from build123d import *

# Parameters (mm, degrees)
SKETCH_1_W          = 44
SKETCH_1_H          = 81
EXTRUDE_1_DEPTH     = 2
SKETCH_12_W         = 12.5
SKETCH_12_H         = 18.4
CUT_EXTRUDE_3_DEPTH = 7.5
SKETCH_15_W         = 1.5
SKETCH_15_H         = 12
EXTRUDE_10_DEPTH    = 8.8
EXTRUDE_11_DEPTH    = 12
EXTRUDE_12_DEPTH    = 12
FILLET_2_R          = 2
FILLET_3_R          = 2
SKETCH_19_R         = 0.85
CUT_EXTRUDE_4_DEPTH = 12
SKETCH_20_R         = 2
CUT_EXTRUDE_5_DEPTH = 1


with BuildPart() as part:
    # 草图1 → 凸台-拉伸1 (new body)
    with BuildSketch(Plane(origin=(0, 0, 0), x_dir=(1, 0, 0), z_dir=(0, 1, 0))):
        with Locations((0, 2.5)):
            Rectangle(SKETCH_1_W, SKETCH_1_H)
    extrude(amount=EXTRUDE_1_DEPTH)

    # 草图12 → 切除-拉伸3 (cut)
    with BuildSketch(Plane.XZ):
        with Locations((9.849848709, 0)):
            Rectangle(SKETCH_12_W, SKETCH_12_H)
    extrude(amount=-CUT_EXTRUDE_3_DEPTH, mode=Mode.SUBTRACT)

    # 草图15 → 凸台-拉伸10 (add)
    with BuildSketch(Plane(origin=(0, 2, 0), x_dir=(1, 0, 0), z_dir=(0, 1, 0))):
        with Locations((2.849848709, 0)):
            Rectangle(SKETCH_15_W, SKETCH_15_H)
        with Locations((16.849848709, 0)):
            Rectangle(SKETCH_15_W, SKETCH_15_H)
    extrude(amount=EXTRUDE_10_DEPTH)

    # 草图16 → 凸台-拉伸11 (add)
    with BuildSketch(Plane.XY.offset(6)):
        Polygon((3.599848709, 10.8), (5.099848709, 8.3), (3.599848709, 8.3), align=None)
    extrude(amount=-EXTRUDE_11_DEPTH)

    # 草图18 → 凸台-拉伸12 (add)
    with BuildSketch(Plane.XY.offset(6)):
        Polygon((16.099848709, 10.8), (14.599848709, 8.3), (16.099848709, 8.3), align=None)
    extrude(amount=-EXTRUDE_12_DEPTH)

    # 圆角2
    fillet_2_edges = [part.edges().sort_by_distance(p)[0] for p in [
        (2.849848709, 2, -6),
        (2.099848709, 2, 0),
        (2.849848709, 2, 6),
        (16.849848709, 2, -6),
        (16.849848709, 2, 6),
        (17.599848709, 2, 0),
    ]]
    fillet(fillet_2_edges, radius=FILLET_2_R)

    # 圆角3
    fillet_3_edges = [part.edges().sort_by_distance(p)[0] for p in [
        (-22, 1, -43),
        (22, 1, -43),
        (22, 1, 38),
        (-22, 1, 38),
    ]]
    fillet(fillet_3_edges, radius=FILLET_3_R)

    # 草图19 → 切除-拉伸4 (cut)
    with BuildSketch(Plane(origin=(0, 2, 0), x_dir=(1, 0, 0), z_dir=(0, 1, 0))):
        with Locations(Location((-19, 40, 0), (0, 0, 270))):
            Circle(SKETCH_19_R)
        with Locations(Location((19, 40, 0), (0, 0, 270))):
            Circle(SKETCH_19_R)
        with Locations(Location((19, -35, 0), (0, 0, 270))):
            Circle(SKETCH_19_R)
        with Locations(Location((-19, -35, 0), (0, 0, 270))):
            Circle(SKETCH_19_R)
    extrude(amount=-CUT_EXTRUDE_4_DEPTH, mode=Mode.SUBTRACT)

    # 草图20 → 切除-拉伸5 (cut)
    with BuildSketch(Plane.XZ):
        with Locations(Location((-19, 35, 0), (0, 0, 270))):
            Circle(SKETCH_20_R)
        with Locations(Location((19, 35, 0), (0, 0, 270))):
            Circle(SKETCH_20_R)
        with Locations(Location((-19, -40, 0), (0, 0, 270))):
            Circle(SKETCH_20_R)
        with Locations(Location((19, -40, 0), (0, 0, 270))):
            Circle(SKETCH_20_R)
    extrude(amount=-CUT_EXTRUDE_5_DEPTH, mode=Mode.SUBTRACT)


solid = part.part
Verification items for the finished model (mm, model axes). A direction names the side the tool comes from. Round coordinates to 2 decimals unless told otherwise and drop trailing zeros. Loops run counter-clockwise (first coordinate to the right, second up) from the corner with the lowest first, then second, coordinate; pieces in that order, holes last. Notation, with made-up numbers: (27.5, 40.25) - (86.5, 40.25) arc R30 ccw to (86.5, 74.25) - close; hole circle Ø3 at (77, 9.25). An arc over 180 degrees is marked (long way). Write item = value, one per line.
Q1. Depth check by flat-ended pin: pin 1 (0.9 mm diameter, centred on x = 16.5, y = 8.5, fed in from +Z); pin 2 (2.5 mm diameter, centred on x = 4, y = 6, fed in from -Z); pin 3 (2.5 mm diameter, centred on x = -19, z = 35, fed in from -Y). Enter the tip coordinate at first touch or a pass-through.
Here are the results:
pin_1 = 6
pin_2 = -6
pin_3 = 1
Q2. Sectioned sample at D-D on y = 3. Record the boundary of the cut face in (x, z), plus the area to 3 significant figures.
Here are the results:
outline = (1.83, -6.27) - (3.6, -6.27) - (3.6, 6.27) - (1.83, 6.27) - close; (16.1, -6.27) - (17.87, -6.27) - (17.87, 6.27) - (16.1, 6.27) - close
area = 44.3 mm^2
Q3. Tool access check on faces 1 (the flat face through (4, 8.3, 0)), 2 (the flat face through (4.34, 9.57, 0.08)), 3 (the flat face through (10, 1, -9.2)). Record the directions out of +Z, -Z, +X, -X, +Y, -Y that give a thin tool (end or side, any length) a straight path to the whole face; none if there is none.
Here are the results:
face_1 = +Z, -Z, -Y
face_2 = +Z, -Z, +Y
face_3 = +Y, -Y
Q4. Material ranges on L1, parallel to X at y = 0.5, z = -40; L2, parallel to X at y = 1.45, z = -40; L3, parallel to X at y = 1.25, z = 5, recorded low to high.
Here are the results:
L1 = -22 to -21, -17 to 17, 21 to 22
L2 = -22 to -19.85, -18.15 to 18.15, 19.85 to 22
L3 = -22 to 3.6, 16.1 to 22
Q5. Sectioned sample at A-A on x = 7. Record the boundary of the cut face in (y, z), plus the area to 3 significant figures.
Here are the results:
outline = (0, -43) - (2, -43) - (2, -9.2) - (0, -9.2) - close; (0, 9.2) - (2, 9.2) - (2, 38) - (0, 38) - close
area = 125 mm^2
Q6. Sectioned sample at B-B on z = -40. Record the boundary of the cut face in (x, y), plus the area to 3 significant figures.
Here are the results:
outline = (-22, 0) - (-21, 0) - (-21, 1) - (-19.85, 1) - (-19.85, 2) - (-22, 2) - close; (-18.15, 1) - (-17, 1) - (-17, 0) - (17, 0) - (17, 1) - (18.15, 1) - (18.15, 2) - (-18.15, 2) - close; (19.85, 1) - (21, 1) - (21, 0) - (22, 0) - (22, 2) - (19.85, 2) - close
area = 76.6 mm^2
Q7. Mould release check, pull along Z, two halves, no side actions. Record for faces 4 (the cylindrical face through (-17.017, 0.493, -39.74)), 5 (the flat face through (0, 0, -3)), 6 (the flat face through (3, 7, 6)): +Z half, -Z half, draft (parallel to the pull), parting line (faces both ways), or undercut.
Here are the results:
face_4 = undercut
face_5 = draft
face_6 = +Z half
Q8. Sectioned sample at C-C on x = -19. Record the boundary of the cut face in (y, z).
Here are the results:
outline = (0, -43) - (2, -43) - (2, -40.85) - (1, -40.85) - (1, -42) - (0, -42) - close; (0, -38) - (1, -38) - (1, -39.15) - (2, -39.15) - (2, 34.15) - (1, 34.15) - (1, 33) - (0, 33) - close; (0, 37) - (1, 37) - (1, 35.85) - (2, 35.85) - (2, 38) - (0, 38) - close
